from build123d import *

# Parameters (mm, degrees)
BOSS_EXTRUDE1_DEPTH = 30
CUT_EXTRUDE1_REACH  = 62.617
SKETCH2_R           = 1


with BuildPart() as part:
    # Sketch1 → Boss-Extrude1 (new body)
    with BuildSketch(Plane(origin=(0, 0, 0), x_dir=(1, 0, 0), z_dir=(0, 1, 0))):
        with BuildLine():
            ThreePointArc((24.385224347, -16), (40.385224347, 0), (24.385224347, 16))
            Line((24.385224347, 16), (-25.838160871, 16))
            ThreePointArc((-25.838160871, 16), (-41.838160871, 0), (-25.838160871, -16))
            Line((-25.838160871, -16), (24.385224347, -16))
        make_face()
        with BuildLine():
            ThreePointArc((-25.838160871, -12.7), (-38.538160871, 0), (-25.838160871, 12.7))
            Line((-25.838160871, 12.7), (24.385224347, 12.7))
            ThreePointArc((24.385224347, 12.7), (37.085224347, 0), (24.385224347, -12.7))
            Line((24.385224347, -12.7), (-25.838160871, -12.7))
        make_face(mode=Mode.SUBTRACT)
    extrude(amount=BOSS_EXTRUDE1_DEPTH)

    # Sketch2 → Cut-Extrude1 (cut, up to next)
    with BuildSketch(Plane.XY.offset(16), mode=Mode.PRIVATE) as cut_extrude1_sk1:
        with Locations((-15.261305548, 27.914958552)):
            Circle(SKETCH2_R)
    cut_extrude1_tool1 = extrude(cut_extrude1_sk1.sketch, amount=-CUT_EXTRUDE1_REACH, mode=Mode.PRIVATE) & part.part
    # Sketch2 → Cut-Extrude1 (cut, up to next)
    with BuildSketch(Plane.XY.offset(16), mode=Mode.PRIVATE) as cut_extrude1_sk2:
        with Locations((10.996521588, 27.914958552)):
            Circle(SKETCH2_R)
    cut_extrude1_tool2 = extrude(cut_extrude1_sk2.sketch, amount=-CUT_EXTRUDE1_REACH, mode=Mode.PRIVATE) & part.part
    add(cut_extrude1_tool1.solids().sort_by_distance((-15.261306, 27.914959, 16))[0], mode=Mode.SUBTRACT)
    add(cut_extrude1_tool2.solids().sort_by_distance((10.996522, 27.914959, 16))[0], mode=Mode.SUBTRACT)


solid = part.part
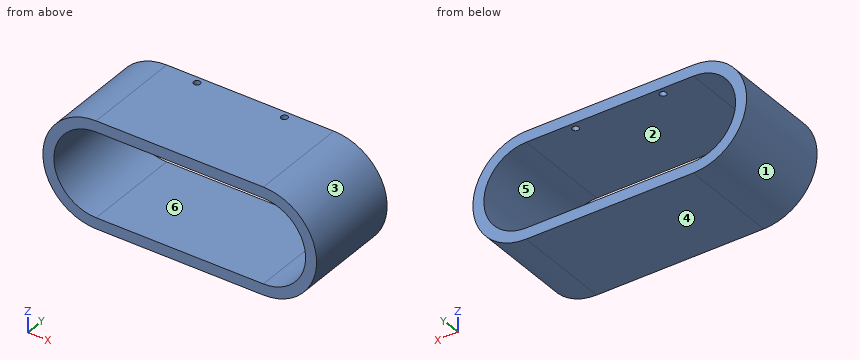
Here's how the part is built. I have some questions about the finished solid (model axes, mm). Face numbers are marked on the shaded views. A direction names the side the tool comes from. Coordinates: 2 decimals unless noted, no trailing zeros. Order: outer loops, then holes, each group sorted by start corner. A loop starts at its lowest first (then second) coordinate and runs counter-clockwise, first axis right, second up. Notation, with made-up numbers: (-17.5, -2.5) -> (17.5, -2.5) arc R17 ccw to (17.5, 27.5) -> close; hole circle Ø10 at (-23.5, -19). An arc over 180 degrees is marked (long way). Answer in a Markdown table with one row per item.
(1) I want a section at C-C on x = -19. List the corners of the cut face in (y, z) for me.
Answer key:
| item | result |
|---|---|
| outline | (0, -16) -> (30, -16) -> (30, -12.7) -> (0, -12.7) -> close; (0, 12.7) -> (30, 12.7) -> (30, 16) -> (0, 16) -> close |
(2) On a 3-axis mill with a long thin cutter (end or side, diameter ignored), from which of +Z, -Z, +X, -X, +Y, -Y can I reach the whole of each face in a straight line? I mean the marked faces 1 and 2. Say none if no direction works.
Answer key:
| item | result |
|---|---|
| face 1 | -X, +Y, -Y |
| face 2 | +Y, -Y |
(3) Will these pins go through, and if not, where does the flat tip stop? pin 1 Ø6 at (y, z) = (4.5, 13) entering from +X; pin 2 Ø2 at (y, z) = (10.5, -8.5) entering from -X; pin 3 Ø2.5 at (x, y) = (11, 27.91) entering from +Z; pin 4 Ø1.8 at (x, y) = (-15.26, 27.91) entering from +Z.
Answer key:
| item | result |
|---|---|
| pin 1 | x = 36.88 |
| pin 2 | x = -39.97 |
| pin 3 | z = 16 |
| pin 4 | z = -12.7 |
(4) I want a section at A-A on y = 25.25. List the corners of the cut face in (x, z) for me, then the cut area to 3 significant figures.
Answer key:
| item | result |
|---|---|
| outline | (-25.84, -16) -> (24.39, -16) arc R16 ccw to (24.39, 16) -> (-25.84, 16) arc R16 ccw to start; hole (-25.84, -12.7) -> (24.39, -12.7) arc R12.7 ccw to (24.39, 12.7) -> (-25.84, 12.7) arc R12.7 ccw to start |
| area | 629 mm^2 |
(5) Thinking about a two-plate mould opening in X: for the marked faces 3, 4, 5 and 6, which applies, +X half, -X half, draft (parallel to the pull), parting line (faces both ways), or undercut?
Answer key:
| item | result |
|---|---|
| face 3 | +X half |
| face 4 | draft |
| face 5 | undercut |
| face 6 | undercut |
(6) Please list where these lines run through material, in increasing order: probe 1 along Z at (x, y) = (13, 20.75); probe 2 along X at (y, z) = (11, -0.5); probe 3 along Z at (x, y) = (32, 4.5).
Answer key:
| item | result |
|---|---|
| probe 1 | -16 to -12.7, 12.7 to 16 |
| probe 2 | -41.83 to -38.53, 37.08 to 40.38 |
| probe 3 | -14.07 to -10.16, 10.16 to 14.07 |
(7) I want a section at B-B on z = 0. List the corners of the cut face in (x, y) for me.
Answer key:
| item | result |
|---|---|
| outline | (-41.84, 0) -> (-38.54, 0) -> (-38.54, 30) -> (-41.84, 30) -> close; (37.09, 0) -> (40.39, 0) -> (40.39, 30) -> (37.09, 30) -> close |
